Design review of the part built by this model. Coordinates are the model's own, in mm. Face numbers are marked on the shaded views. A direction names the side the tool comes from. Give positions to 0.01 mm unless a question says otherwise; leave off trailing zeros. Order: outer loops, then holes, each group sorted by start corner. A loop starts at its lowest first (then second) coordinate and runs counter-clockwise, first axis right, second up. Notation, with made-up numbers: M -7.5,62 L 20.5,62 A19 cw 20.5,88 Z; hole C 57,-8 d10. An arc over 180 degrees is marked long. Answer as a JSON object with one key per item and string values.
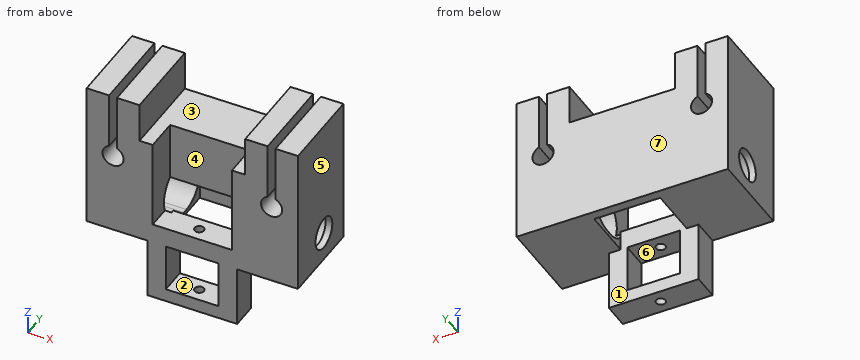
Autodesk Inventor part; units mm, degrees
ref_plane "Work Plane5" through (-40, 21.062, -10) normal (-1, 0, 0) x (0, 0, 1)
ref_plane "YZ Plane" through (0, 0, 0) normal (1, 0, 0) x (0, 1, 0)
ref_plane "XZ Plane" through (0, 0, 0) normal (0, 1, 0) x (-1, 0, 0)
sketch "Sketch1" plane through (0, 0, 0) normal (0, 1, 0) x (-1, 0, 0)
  arc A0 (8.5, 13.7081) -> (11.5, 13.7081) centre (10, 10) ccw
  line L0 (8.5, 20) -> (8.5, 13.7081)
  line L1 (11.5, 20) -> (11.5, 13.7081)
  line L2 (10, 20) -> (10, 18.7339)
  line L3 (20, 20) -> (10, 20)
  line L4 (8.5, 20) -> (0, 20)
  line L5 (0, 20) -> (0, 0)
  line L6 (0, 0) -> (20, 0)
  line L7 (20, 0) -> (20, 20)
  arc A1 (68.5, 13.7081) -> (71.5, 13.7081) centre (70, 10) ccw
  line L8 (68.5, 20) -> (68.5, 13.7081)
  line L9 (71.5, 20) -> (71.5, 13.7081)
  line L10 (70, 20) -> (70, 18.3732)
  line L11 (80, 20) -> (70, 20)
  line L12 (68.5, 20) -> (60.9559, 20)
  line L13 (60.9559, 20) -> (60.9559, 0)
  line L14 (60.9559, 0) -> (80, 0)
  line L15 (80, 0) -> (80, 20)
  line L16 (60.9559, 0) -> (20, 0)
  line L17 (20, 0) -> (20, 20)
  line L18 (20, 20) -> (60.9559, 20)
  line L19 (60.9559, 20) -> (60.9559, 0)
  dimension "d2" = 8
  dimension "d7" = 1.5
  dimension "d8" = 1.5
  dimension "d16" = 10
  dimension "d17" = 8
  dimension "d18" = 1.5
  dimension "d19" = 1.5
  dimension "d20" = 10
  dimension "d22" = 80
  dimension "d23" = 10
  dimension "d24" = 0
  dimension "d25" = 60
  dimension "d26" = 20
  dimension "d27" = 20
  dimension "d28" = 20
  dimension "d29" = 20
  dimension "d30" = 10
  dimension "d31" = 10
  dimension "d32" = 20
extrude "Extrusion1" add sketch "Sketch1" along normal blind 36
sketch "Sketch5" plane through (-80, 0, 0) normal (-1, 0, 0) x (0, 0, 1)
  line L0 (20, 0) -> (20, 36)
  line L1 (20, 36) -> (-15, 36)
  line L2 (-15, 6) -> (20, 6)
  line L3 (20, 6) -> (20, 36)
  line L4 (-15, 36) -> (-15, 29.1398)
  line L5 (-15, 12.9843) -> (-15, 6)
  line L6 (0, 0) -> (0, 36)
  line L7 (0, 0) -> (0, 36)
  line L8 (0, 6) -> (0, 36)
  arc A0 (-15, 12.9843) -> (-15, 29.1398) centre (-10, 21.062) ccw
  dimension "d40" = 30
  dimension "d41" = 35
  dimension "d45" = 20
  dimension "d85" = 19
  dimension "d86" = 5
  dimension "d87" = 15
extrude "Extrusion5" add sketch "Sketch5" against normal blind 80 contours L2 L5 A0 L4 L1 L6
sketch "Sketch13" plane through (0, 36, 0) normal (0, 1, 0) x (1, 0, 0)
  line L0 (-80, -20) -> (-80, 15)
  line L1 (-80, -20) -> (-71.5, -20)
  line L2 (-71.5, -20) -> (-71.5, -13.7081)
  arc A0 (-68.5, -13.7081) -> (-71.5, -13.7081) centre (-70, -10) ccw
  line L3 (-68.5, -13.7081) -> (-68.5, -20)
  line L4 (-68.5, -20) -> (-11.5, -20)
  line L5 (-11.5, -20) -> (-11.5, -13.7081)
  arc A1 (-8.5, -13.7081) -> (-11.5, -13.7081) centre (-10, -10) ccw
  line L6 (-8.5, -13.7081) -> (-8.5, -20)
  line L7 (-8.5, -20) -> (0, -20)
  line L8 (0, -20) -> (0, 15)
  line L9 (-80, 15) -> (0, 15)
  point P0 (0, 0)
extrude "Extrusion11" cut sketch "Sketch13" against normal blind 1
sketch "Sketch16" plane through (-80, 6, -15) normal (0, 0, -1) x (-1, 0, 0)
  line L0 (-80, -6) -> (0, -6)
  line L1 (0, 6.9843) -> (-80, 6.9843)
  line L2 (-80, -6) -> (0, -6)
  line L3 (0, -6) -> (0, 6.9843)
  line L4 (0, 6.9843) -> (-80, 6.9843)
  line L5 (-80, 6.9843) -> (-80, -6)
  line L6 (0, -6) -> (0, 29)
  line L7 (0, 23.1398) -> (-80, 23.1398)
  line L8 (0, 29) -> (-80, 29)
  line L9 (-80, 29) -> (-80, 23.1398)
  line L10 (-80, 23.1398) -> (0, 23.1398)
  line L11 (0, 23.1398) -> (0, 29)
extrude "Extrusion13" add sketch "Sketch16" along normal blind 6
sketch "Sketch17" plane through (0, 0, 0) normal (0, 0, -1) x (-1, 0, 0)
  line L0 (80, 6) -> (0, 6)
  line L1 (0, 0) -> (80, 0)
  line L2 (80, 6) -> (0, 6)
  line L3 (80, 6) -> (80, 0)
  line L4 (0, 6) -> (0, 0)
extrude "Extrusion14" add sketch "Sketch17" along normal blind 20
sketch "Sketch18" plane through (-68.5, 0, 20) normal (0, 0, 1) x (1, 0, 0)
  line L0 (13.5, 0) -> (43.5, 0)
  line L1 (43.5, 0) -> (43.5, 15)
  line L2 (43.5, 15) -> (13.5, 15)
  line L3 (13.5, 15) -> (13.5, 0)
  line L4 (-11.5, 0) -> (-11.5, 35)
  line L5 (0, 0) -> (57, 0)
  point P0 (68.5, 0)
  dimension "d107" = 30
  dimension "d108" = 25
  dimension "d109" = 15
  dimension "d110" = 0
extrude "Extrusion15" cut sketch "Sketch18" against normal blind 37
sketch "Sketch19" plane through (0, 0, 0) normal (0, -1, 0) x (1, 0, 0)
  line L0 (-80, -21) -> (0, -21)
  line L1 (-30, -21) -> (-23, -21)
  line L2 (-23, -21) -> (-23, -44)
  line L3 (-23, -44) -> (-30, -44)
  line L4 (-30, -44) -> (-30, -21)
  line L5 (-30, -44) -> (-50, -44)
  line L6 (-50, -44) -> (-50, -39)
  line L7 (-50, -39) -> (-30, -39)
  line L8 (-30, -39) -> (-30, -44)
  line L9 (-50, -44) -> (-57, -44)
  line L10 (-57, -44) -> (-57, -21)
  line L11 (-57, -21) -> (-50, -21)
  line L12 (-50, -21) -> (-50, -44)
  line L13 (0, -21) -> (0, 20)
  point P0 (0, 0)
  dimension "d113" = 7
  dimension "d114" = 7
  dimension "d115" = 5
  dimension "d116" = 18
  dimension "d117" = 20
  dimension "d118" = 23
extrude "Extrusion16" add sketch "Sketch19" against normal blind 15.5 contours L0 L12 L6 L9 L10 | L0 L2 L3 L4 | L7 L4 L5 L6
sketch "Sketch20" plane through (-23, 0, -44) normal (0, 0, -1) x (-1, 0, 0)
  circle A0 centre (17, 7.5) radius 1.75
  line L0 (34, 0) -> (0, 0)
  line L1 (-23, 12.9843) -> (-23, 0)
  dimension "d121" = 3.5
  dimension "d122" = 7.5
  dimension "d123" = 40
extrude "Extrusion17" cut sketch "Sketch20" against normal blind 80
sketch "Sketch21" plane through (0, 0, 0) normal (0, -1, 0) x (1, 0, 0)
  line L0 (0, -0.5) -> (-80, -0.5)
  line L1 (0, -21) -> (-23, -21)
  line L2 (0, -21) -> (0, 20)
  line L3 (0, 20) -> (-8.5, 20)
  line L4 (-8.5, 20) -> (-8.5, 13.7081)
  arc A0 (-11.5, 13.7081) -> (-8.5, 13.7081) centre (-10, 10) ccw
  line L5 (-11.5, 13.7081) -> (-11.5, 20)
  line L6 (-25, 20) -> (-11.5, 20)
  line L7 (-25, 20) -> (-25, -17)
  line L8 (-25, -17) -> (-55, -17)
  line L9 (-55, -17) -> (-55, 20)
  line L10 (-68.5, 20) -> (-55, 20)
  line L11 (-68.5, 13.7081) -> (-68.5, 20)
  arc A1 (-71.5, 13.7081) -> (-68.5, 13.7081) centre (-70, 10) ccw
  line L12 (-71.5, 20) -> (-71.5, 13.7081)
  line L13 (-80, 20) -> (-71.5, 20)
  line L14 (-80, 20) -> (-80, -21)
  line L15 (-57, -21) -> (-80, -21)
  line L16 (-57, -21) -> (-57, -44)
  line L17 (-57, -44) -> (-23, -44)
  line L18 (-23, -44) -> (-23, -21)
  line L19 (-30, -21) -> (-30, -39)
  line L20 (-30, -39) -> (-50, -39)
  line L21 (-50, -39) -> (-50, -21)
  line L22 (-30, -21) -> (-50, -21)
  point P0 (0, 0)
extrude "Extrusion18" cut sketch "Sketch21" against normal blind 2.5 contours L2 L1 L18 L17 L16 L15 L14 L0 L9 L8 L7 | L0 L7 L6 L5 A0 L4 L3 L2 | L0 L14 L13 L12 A1 L11 L10 L9 | L19 L20 L21 L22
ref_plane "Work Plane5" through (-40, 21.062, -10) normal (-1, 0, 0) x (0, 0, 1)
sketch "Sketch25" plane through (-80, 6, -21) normal (0, 0, -1) x (-1, 0, 0)
  line L0 (-80, 6.9843) -> (-80, -3.5)
  line L1 (0, 29) -> (-80, 29)
  line L2 (-80, -3.5) -> (-52.5, -3.5)
  line L3 (-52.5, -3.5) -> (-52.5, 29)
  line L4 (-52.5, 29) -> (-80, 29)
  line L5 (-80, 29) -> (-80, -3.5)
  line L6 (0, 23.1398) -> (0, 29)
  line L7 (0, 29) -> (-27.5, 29)
  line L8 (-27.5, 29) -> (-27.5, -1)
  line L9 (-27.5, -1) -> (0, -1)
  line L10 (0, -1) -> (0, 29)
  point P0 (-80, -6)
  dimension "d138" = 27.5
  dimension "d139" = 27.5
  dimension "d140" = 30
extrude "Extrusion21" add sketch "Sketch25" against normal blind 7.5
sketch "Sketch22" plane through (-40, 21.062, -10) normal (-1, 0, 0) x (0, 0, 1)
  arc A0 (-9.4999, -0.9509) -> (9.4999, -0.9509) centre (0, -1) ccw
  arc A1 (9.4999, 0.9509) -> (-9.4999, 0.9509) centre (0, 1) ccw
  line L0 (9.4999, -0.9509) -> (9.4999, 1.0491)
  line L1 (-9.4999, -0.9509) -> (-9.4999, 1.0491)
  point P0 (0, 0)
  dimension "d170" = 1
  dimension "d171" = 1
  dimension "d172" = 19
  dimension "d173" = 19
extrude "Extrusion19" cut sketch "Sketch22" along normal mid plane 75
sketch "Sketch24" plane through (-80, 6, -21) normal (0, 0, -1) x (-1, 0, 0)
  line L0 (0, 29) -> (-80, 29)
  line L1 (-27.5, 29) -> (-52.5, 29)
  line L2 (-52.5, 29) -> (-52.5, 4.062)
  line L3 (-52.5, 4.062) -> (-27.5, 4.062)
  line L4 (-27.5, 4.062) -> (-27.5, 29)
  line L5 (0, 23.1398) -> (0, 29)
  line L6 (-80, 6.9843) -> (-80, -3.5)
  line L7 (-52.5, 29) -> (-80, 29)
  line L8 (-80, 29) -> (-80, -3.5)
  line L9 (-80, -3.5) -> (-52.5, -3.5)
  line L10 (-52.5, -3.5) -> (-52.5, 29)
  line L11 (0, -3.5) -> (0, 6.9843)
  line L12 (-27.5, 29) -> (0, 29)
  line L13 (0, 29) -> (0, -3.5)
  line L14 (0, -3.5) -> (-27.5, -3.5)
  line L15 (-27.5, -3.5) -> (-27.5, 29)
  line L16 (-27.5, 25.5) -> (-52.5, 25.5)
  line L17 (-52.5, 25.5) -> (-52.5, 6.5)
  line L18 (-52.5, 6.5) -> (-27.5, 6.5)
  line L19 (-27.5, 6.5) -> (-27.5, 25.5)
  line L20 (-77.5, 25.562) -> (-2.5, 25.562)
  point P0 (-80, -6)
  point P1 (-52.5, 6.5)
  point P2 (-27.5, 6.5)
  point P3 (-27.5, 25.5)
  point P4 (-52.5, 25.5)
  dimension "d133" = 25
  dimension "d134" = 27.5
  dimension "d174" = 3.5
  dimension "d175" = 19
extrude "Extrusion20" cut sketch "Sketch24" against normal blind 10 contours L4 L18 L2 L16
sketch "Sketch26" plane through (0, 35, 20) normal (1, 0, 0) x (0, 0, -1)
  arc A0 (33.5, -5.1062) -> (33.5, -22.7697) centre (30, -13.938) ccw
  circle A1 centre (30, -13.938) radius 6
  line L0 (41, 0) -> (41, -32.5)
  line L1 (0, 0) -> (41, 0)
  line L2 (0, -32.5) -> (0, 0)
  line L3 (0, -32.5) -> (41, -32.5)
  line L4 (33.5, -22.7697) -> (33.5, -5.1062)
  arc A2 (33.5, -5.1062) -> (33.5, -22.7697) centre (30, -13.938) ccw
  point P0 (20, -35)
  point P1 (35, -8.3478)
  point P2 (35, -19.5282)
  dimension "d143" = 12
extrude "Extrusion22" add sketch "Sketch26" against normal blind 2.5 contours L4 A1 A0
sketch "Sketch27" plane through (-80, 35, -21) normal (-1, 0, 0) x (0, 0, 1)
  arc A0 (7.5, -22.7697) -> (7.5, -5.1062) centre (11, -13.938) ccw
  line L0 (7.5, -5.1062) -> (7.5, -22.7697)
  line L1 (0, -32.5) -> (0, 0)
  line L2 (0, -32.5) -> (41, -32.5)
  line L3 (41, -32.5) -> (41, 0)
  line L4 (41, 0) -> (0, 0)
  circle A1 centre (11, -13.938) radius 6
  point P0 (21, -35)
extrude "Extrusion23" add sketch "Sketch27" against normal blind 2.5 contours L0 A1 A0
sketch "Sketch28" plane through (-80, 6, -21) normal (0, 0, -1) x (-1, 0, 0)
  line L0 (-77.5, 23.062) -> (-2.5, 23.062)
  line L1 (-57.32, 23.062) -> (-20.6249, 23.062)
  line L2 (-20.6249, 23.062) -> (-20.6249, 8)
  line L3 (-20.6249, 8) -> (-57.32, 8)
  line L4 (-57.32, 8) -> (-57.32, 23.062)
  line L5 (-57, 9.5) -> (-23, 9.5)
  point P0 (-80, -6)
  dimension "d152" = 1.5
extrude "Extrusion24" cut sketch "Sketch28" along normal blind 30.5
sketch "Sketch29" plane through (-80, 35, -21) normal (-1, 0, 0) x (0, 0, 1)
  arc A0 (7.5, -18.8114) -> (7.5, -9.0646) centre (11, -13.938) ccw
  circle A1 centre (11, -13.938) radius 6
  point P0 (21, -35)
  point P1 (7.5, -9.0646)
  point P2 (7.5, -18.8114)
extrude "Extrusion25" cut sketch "Sketch29" against normal blind 100.5
sketch "Sketch30" plane through (-68.5, 35, 20) normal (0, 0, 1) x (1, 0, 0)
  line L0 (-11.5, -32.5) -> (-3, -32.5)
  line L1 (-3, -32.5) -> (-3, 0)
  line L2 (-3, 0) -> (-11.5, 0)
  line L3 (-11.5, -32.5) -> (-11.5, 0)
  line L4 (0, -32.5) -> (13.5, -32.5)
  line L5 (13.5, -32.5) -> (13.5, -20)
  line L6 (13.5, -20) -> (43.5, -20)
  line L7 (43.5, -20) -> (43.5, -32.5)
  line L8 (43.5, -32.5) -> (57, -32.5)
  line L9 (57, -32.5) -> (57, 0)
  line L10 (57, 0) -> (0, 0)
  line L11 (0, -32.5) -> (0, 0)
  line L12 (60, -32.5) -> (68.5, -32.5)
  line L13 (68.5, -32.5) -> (68.5, 0)
  line L14 (68.5, 0) -> (60, 0)
  line L15 (60, -32.5) -> (60, 0)
  point P0 (68.5, -35)
extrude "Extrusion26" add sketch "Sketch30" along normal blind 15
sketch "Sketch31" plane through (-68.5, 35, 35) normal (0, 0, 1) x (1, 0, 0)
  line L0 (-11.5, 0) -> (68.5, 0)
  line L1 (43.5, -32.5) -> (57, -32.5)
  line L2 (8.5, 0) -> (50.25, 0)
  line L3 (50.25, 0) -> (50.25, -32.5)
  line L4 (50.25, -32.5) -> (8.5, -32.5)
  line L5 (8.5, -32.5) -> (8.5, 0)
  line L6 (-11.5, 0) -> (-11.5, -32.5)
  line L7 (48.5, -32.5) -> (48.5, 0)
  line L8 (68.5, -32.5) -> (68.5, 0)
  point P0 (68.5, -35)
  dimension "d157" = 20
  dimension "d158" = 20
extrude "Extrusion27" cut sketch "Sketch31" against normal blind 15 contours L0 L7 L1 L4 L5
sketch "Sketch32" plane through (-68.5, 0, -17) normal (0, 0, 1) x (1, 0, 0)
  line L0 (38.5, 12.5) -> (38.5, 2.5)
  line L1 (16, 12.5) -> (16, 5)
  line L2 (16, 5) -> (13.5, 5)
  line L3 (13.5, 2.5) -> (13.5, 5)
  line L4 (13.5, 2.5) -> (41, 2.5)
  line L5 (41, 2.5) -> (41, 12.5)
  circle A0 centre (28.5, 7.5) radius 1.75
  line L6 (41, 12.5) -> (16, 12.5)
  point P0 (68.5, 0)
  point P1 (38.5, 14)
  point P2 (38.5, 12.9843)
extrude "Extrusion28" add sketch "Sketch32" along normal up to surface (3.5 mm away)
sketch "Sketch33" plane through (-27.5, 14, -21) normal (0, 1, 0) x (1, 0, 0)
  line L0 (-2.5, 0) -> (-2.5, 18)
  line L1 (0, 0) -> (-2.5, 0)
  line L2 (4.5, 0) -> (0, 0)
  line L3 (4.5, 23) -> (4.5, 0)
  line L4 (-29.5, 23) -> (4.5, 23)
  line L5 (-29.5, 0) -> (-29.5, 23)
  line L6 (-25, 0) -> (-29.5, 0)
  line L7 (-22.5, 0) -> (-25, 0)
  line L8 (-22.5, 18) -> (-22.5, 0)
  line L9 (-2.5, 18) -> (-22.5, 18)
  point P0 (27.5, -21)
extrude "Extrusion29" cut sketch "Sketch33" against normal blind 1.5
equation "\"d2\" = RodDiameter"
equation "\"d17\" = d2"
equation "\"d85\" = XLinearBearingOD"
equation "\"d139\" = d138"
equation "\"d172\" = XLinearBearingOD"
equation "\"d173\" = XLinearBearingOD"
equation "\"d175\" = XLinearBearingOD"
equation "\"RodDiameter\" = 8"
equation "\"VerticalBearingOD\" = 16"
equation "\"PrintingClearance\" = 0.2"
equation "\"d21\" = 8"
equation "\"TubeID\" = 18"
equation "\"XLinearBearingOD\" = 19"
properties part number "GantryHolder" material "PET Plastic"
(1) Draft analysis for pull direction X (two halves, no side actions). For the marked faces 5, 6 and 7, state which applies: +X half, -X half, draft (parallel to the pull), parting line (faces both ways), or undercut.
Checked values:
{"face 5": "+X half", "face 6": "undercut", "face 7": "draft"}
(2) Tool access review of the marked faces 1, 2, 3 and 4: name each direction out of +Z, -Z, +X, -X, +Y, -Y from which nothing blocks a thin tool from reaching the whole face with its end or side.
Checked values:
{"face 1": "-Z", "face 2": "+Y, -Y", "face 3": "+Z, +Y, -Y", "face 4": "+Z, -Y"}
(3) We need section C-C (z = 10). Write out the cut boundary in (x, y), plus the area to 4 significant figures.
Checked values:
{"outline": "M -80,2.5 L -74,2.5 L -74,35 L -80,35 Z; M -66,2.5 L -55,2.5 L -55,15 L -25,15 L -25,2.5 L -14,2.5 L -14,35 L -66,35 Z; M -6,2.5 L 0,2.5 L 0,35 L -6,35 Z", "area": "1,705 mm^2"}
(4) We need section B-B (x = -59). Write out the cut boundary in (y, z).
Checked values:
{"outline": "M 2.5,-21 L 35,-21 L 35,20 L 2.5,20 Z; hole M 20.11,-19.5 L 22.01,-19.5 A9.5 ccw long 22.01,-0.5 L 20.11,-0.5 A9.5 ccw long Z"}
(5) Insertion check: pin 1 (2 mm diameter, centred on x = -40, y = 7.5, fed in from +Z); pin 2 (1 mm diameter, centred on x = -42, z = 16.5, fed in from -Y); pin 3 (11 mm diameter, centred on x = -34.5, y = 6, fed in from +Z); pin 4 (8 mm diameter, centred on y = 8.5, z = -32.5, fed in from +X). Each pin has a flat end and moves straight along its axis. Give the tip position at first contact, or say it passes through.
Checked values:
{"pin 1": "passes through", "pin 2": "stops at y = 15", "pin 3": "stops at z = -13.5", "pin 4": "stops at x = -23"}
(6) To check wall thickness, follow L1, parallel to X at y = 8.5, z = 31.5; L2, parallel to Y at x = -40, z = -15; L3, parallel to X at y = 11, z = 17.5. State the ranges of each line that lie inside material, in increasing order. Write a range as from..to.
Checked values:
{"L1": "x = -80..-71.5, -68.5..-60, -20..-11.5, -8.5..0", "L2": "y = 2.5..5.75, 9.25..12.5, 31.5..35", "L3": "x = -80..-71.5, -68.5..-55, -25..-11.5, -8.5..0"}
(7) We need section D-D (y = 18). Count the separate pieces of the cut face and the enclosed holes in it, plus the area to 3 significant figures.
Checked values:
{"separate pieces": "3", "enclosed holes": "0", "area": "2,170 mm^2"}
(8) We need section A-A (z = -22). Write out the cut boundary in (x, y), plus the area to 3 significant figures.
Checked values:
{"outline": "M -57,2.5 L -50,2.5 L -50,12.5 L -57,12.5 Z; M -30,2.5 L -23,2.5 L -23,12.5 L -30,12.5 Z", "area": "140 mm^2"}
